```python
from build123d import *

# Parameters (mm, degrees)
EXTRUDE1_DEPTH          = 5.334
SKETCH20_W              = 5.08
SKETCH20_H              = 5.715
EXTRUDE3_DEPTH          = 12.7
SKETCH22_W              = 0.889
SKETCH22_H              = 2.54
EXTRUDE5_DEPTH          = 5.334
SKETCH23_W              = 5.08
SKETCH23_H              = 1.5875
EXTRUDE6_DEPTH          = 3.683
FILLET5_R               = 1.6002
FILLET6_R               = 0.8382
FILLET2_R               = 0.762
CUT_EXTRUDE4_DEPTH      = 1
CUT_EXTRUDE4_DEPTH_BACK = 11.922
CUT_EXTRUDE5_DEPTH      = 1
CUT_EXTRUDE5_DEPTH_BACK = 11.922
CUT_EXTRUDE7_DEPTH      = 1
CUT_EXTRUDE7_DEPTH_BACK = 11.922
CUT_EXTRUDE8_DEPTH      = 1
CUT_EXTRUDE8_DEPTH_BACK = 18.78
BOSS_EXTRUDE1_DEPTH     = 7.366


with BuildPart() as part:
    # Sketch2 → Extrude1 (new body)
    with BuildSketch(Plane.XY):
        Polygon((-5.08, 0), (-5.08, -1.524), (0, -1.524), (0, 0), (0, 9.398), (-25.4, 9.398), (-25.4, 0), align=None)
    extrude(amount=EXTRUDE1_DEPTH)

    # Sketch20 → Extrude3 (add)
    with BuildSketch(Plane.XY.offset(5.334)):
        with Locations((-2.54, 6.5405)):
            Rectangle(SKETCH20_W, SKETCH20_H)
    extrude(amount=EXTRUDE3_DEPTH)

    # Sketch22 → Extrude5 (add)
    with BuildSketch(Plane.XY.offset(5.334)):
        with Locations((-25.8445, 8.128)):
            Rectangle(SKETCH22_W, SKETCH22_H)
    extrude(amount=-EXTRUDE5_DEPTH)

    # Sketch23 → Extrude6 (add)
    with BuildSketch(Plane.XZ.offset(-3.683)):
        with Locations((-2.54, 17.24025)):
            Rectangle(SKETCH23_W, SKETCH23_H)
    extrude(amount=EXTRUDE6_DEPTH)

    # Fillet5
    fillet5_edges = [part.edges().sort_by_distance(p)[0] for p in [
        (-26.289, 8.128, 5.334),
    ]]
    fillet(fillet5_edges, radius=FILLET5_R)

    # Fillet6
    fillet6_edges = [part.edges().sort_by_distance(p)[0] for p in [
        (-5.08, 1.8415, 16.4465),
    ]]
    fillet(fillet6_edges, radius=FILLET6_R)

    # Fillet2
    fillet2_edges = [part.edges().sort_by_distance(p)[0] for p in [
        (-5.08, 6.5405, 5.334),
        (0, 4.699, 18.034),
        (-5.08, 4.699, 18.034),
        (0, 1.0795, 5.334),
    ]]
    fillet(fillet2_edges, radius=FILLET2_R)

    # Sketch26 → Cut-Extrude4 (cut, two sides)
    with BuildSketch(Plane(origin=(0, 9.398, 0), x_dir=(1, 0, 0), z_dir=(0, 1, 0))) as cut_extrude4_sk:
        Polygon((20.812608211, 70.762867918), (0, 0), (-5.08, -17.272), (-25.892608211, -88.034867918), (115.633127624, -129.66008434), (162.338344046, 29.137651496), align=None)
    extrude(amount=CUT_EXTRUDE4_DEPTH, mode=Mode.SUBTRACT)
    extrude(cut_extrude4_sk.sketch, amount=-CUT_EXTRUDE4_DEPTH_BACK, mode=Mode.SUBTRACT)

    # Sketch27 → Cut-Extrude5 (cut, two sides)
    with BuildSketch(Plane(origin=(0, 9.398, 0), x_dir=(1, 0, 0), z_dir=(0, 1, 0))) as cut_extrude5_sk:
        Polygon((-68.071537779, -14.906771648), (-5.08, -14.906771648), (-4.384344602, -14.906771648), (58.607193177, -14.906771648), (58.607193177, -140.889847207), (-68.071537779, -140.889847207), align=None)
    extrude(amount=CUT_EXTRUDE5_DEPTH, mode=Mode.SUBTRACT)
    extrude(cut_extrude5_sk.sketch, amount=-CUT_EXTRUDE5_DEPTH_BACK, mode=Mode.SUBTRACT)

    # Sketch28 → Cut-Extrude7 (cut, two sides)
    with BuildSketch(Plane(origin=(0, 9.398, 0), x_dir=(1, 0, 0), z_dir=(0, 1, 0))) as cut_extrude7_sk:
        Polygon((-17.78, 56.40432053), (-17.78, 0), (-17.78, -5.334), (-17.78, -61.73832053), (-130.588641061, -61.73832053), (-130.588641061, 56.40432053), align=None)
    extrude(amount=CUT_EXTRUDE7_DEPTH, mode=Mode.SUBTRACT)
    extrude(cut_extrude7_sk.sketch, amount=-CUT_EXTRUDE7_DEPTH_BACK, mode=Mode.SUBTRACT)

    # Sketch29 → Cut-Extrude8 (cut, two sides)
    with BuildSketch(Plane.ZY.offset(17.78)) as cut_extrude8_sk:
        Polygon((-42.326728478, 3.1496), (0, 3.1496), (5.334, 3.1496), (47.660728478, 3.1496), (47.660728478, -81.503856957), (-42.326728478, -81.503856957), align=None)
    extrude(amount=CUT_EXTRUDE8_DEPTH, mode=Mode.SUBTRACT)
    extrude(cut_extrude8_sk.sketch, amount=-CUT_EXTRUDE8_DEPTH_BACK, mode=Mode.SUBTRACT)

    # Sketch30 → Boss-Extrude1 (add)
    with BuildSketch(Plane(origin=(0, 9.398, 0), x_dir=(1, 0, 0), z_dir=(0, 1, 0))):
        Polygon((-5.08, -14.906771648), (-5.08, 0), (0, 0), (-4.384344602, -14.906771648), align=None)
    extrude(amount=-BOSS_EXTRUDE1_DEPTH)


solid = part.part
```
Geometry: final body of the model. Coordinates: model frame, mm. A direction names the side the tool comes from. Round coordinates to 2 decimals unless told otherwise and drop trailing zeros. Order: outer loops, then holes, each group sorted by start corner. A loop starts at its lowest first (then second) coordinate and runs counter-clockwise, first axis right, second up. Notation, with made-up numbers: (32, -17) -> (49, -17) arc R36 cw to (49, 20) -> close; hole circle Ø5 at (66, 88). An arc over 180 degrees is marked (long way). Use one line per item in the form item = value.
(1) Access query for faces 3 (the face through (-12, 3.15, 3)), 4 (the face through (-9, 9.398, 4)). Directions: +Z, -Z, +X, -X, +Y, -Y. A direction counts if a zero-diameter tool reaches every point of the face in a straight line with its end or side. Return the directions, or none.
Results list:
face_3 = +Z, -Z, -X, -Y
face_4 = +Z, -Z, +X, -X, +Y
(2) First-contact query: pin 1 Ø2 at (x, y) = (-4, 5.5) entering from -Z; pin 2 Ø4 at (x, y) = (-15.5, 3) entering from +Z; pin 3 Ø6 at (x, z) = (-11, 2.5) entering from -Y. Flat tips, straight axial feed; report the tip coordinate or a pass-through.
Results list:
pin_1 = 0
pin_2 = 5.33
pin_3 = 3.15
(3) Section D-D on x = -2.75. Return loops of the section in (y, z).
Results list:
outline = (2.03, 0) -> (9.4, 0) -> (9.4, 9.35) -> (2.03, 9.35) -> close
(4) Draft query along X for faces 1 (the face through (-17.78, 6, 3)), 2 (the face through (-9, 6, 0)). Return one class per face: pulls with the +X half, pulls with the -X half, needs draft (parallel to the pull), parting line crosses it, or undercut.
Results list:
face_1 = pulls with the -X half
face_2 = needs draft
(5) Section C-C on x = -7.5. Return loops of the section in (y, z).
Results list:
outline = (3.15, 0) -> (9.4, 0) -> (9.4, 5.33) -> (3.15, 5.33) -> close
(6) Section A-A on z = 2.75. Return loops of the section in (x, y).
Results list:
outline = (-17.78, 3.15) -> (-5.08, 3.15) -> (-5.08, 2.03) -> (-0.81, 2.03) -> (-0.81, 9.4) -> (-17.78, 9.4) -> close
(7) Ray query, probe 1 along Y at (x, z) = (-11.5, 4); probe 2 along Z at (x, y) = (-16, 7.5); probe 3 along X at (y, z) = (5, 2). Return the intervals inside material, ascending. Write a range as [from, to].
Results list:
probe_1 = [3.15, 9.4]
probe_2 = [0, 5.33]
probe_3 = [-17.78, -0.59]
(8) Section B-B on y = 5. Return loops of the section in (x, z), and give its area (3 significant figures).
Results list:
outline = (-17.78, 0) -> (0, 0) -> (-4.38, 14.91) -> (-5.08, 14.91) -> (-5.08, 6.1) arc R0.76 cw to (-5.84, 5.33) -> (-17.78, 5.33) -> close
area = 111 mm^2
